Can you work these out from the model? Positions are in its coordinate system, mm. A direction names the side the tool comes from. Coordinates: 2 decimals unless noted, no trailing zeros. Loops run counter-clockwise (first coordinate to the right, second up) from the corner with the lowest first, then second, coordinate; pieces in that order, holes last.
```python
from build123d import *

# Parameters (mm, degrees)
ESQUISSE1_W             = 10
ESQUISSE1_H             = 15
BOSS_EXTRU_1_DEPTH      = 10
CONG_1_RADIUS           = 5
CONG_1_LENGTH           = 10
ESQUISSE3_W             = 5
ESQUISSE3_H             = 12
ENL_V_MAT_EXTRU_1_DEPTH = 10
ESQUISSE4_W             = 10
ESQUISSE4_H             = 10
BOSS_EXTRU_2_DEPTH      = 3
ESQUISSE5_R             = 1
ENL_V_MAT_EXTRU_2_DEPTH = 3
ESQUISSE6_R             = 2
ENL_V_MAT_EXTRU_3_DEPTH = 21.862646045
CONG_2_R                = 0.5
CONG_3_R                = 0.5


with BuildPart() as part:
    # Esquisse1 → Boss.-Extru.1 (new body)
    with BuildSketch(Plane.XY):
        Rectangle(ESQUISSE1_W, ESQUISSE1_H)
    extrude(amount=BOSS_EXTRU_1_DEPTH)

    # Congé1: full round fillet: the end face becomes a half cylinder, R = half its width
    cong_1_face = Plane((0, -7.5, 5), x_dir=(0, 0, 1), z_dir=(0, -1, 0))  # on the end face: x along it, z out of the body
    cong_1_slab = cong_1_face.offset(-CONG_1_RADIUS / 2) * Box(CONG_1_LENGTH, 2 * CONG_1_RADIUS, CONG_1_RADIUS, mode=Mode.PRIVATE)  # the body's end, R deep
    cong_1_round = Plane((0, -2.5, 5), x_dir=(0, -1, 0), z_dir=(0, 0, 1)) * Cylinder(CONG_1_RADIUS, CONG_1_LENGTH, mode=Mode.PRIVATE)  # its axis R under the face
    add(cong_1_slab - cong_1_round, mode=Mode.SUBTRACT)

    # Esquisse3 → Enlèv. mat.-Extru.1 (cut)
    with BuildSketch(Plane.ZY.offset(5)):
        with Locations((5, -1.5)):
            Rectangle(ESQUISSE3_W, ESQUISSE3_H)
    extrude(amount=-ENL_V_MAT_EXTRU_1_DEPTH, mode=Mode.SUBTRACT)

    # Esquisse4 → Boss.-Extru.2 (add)
    # profile 1 of 2: a face of its own
    with BuildSketch(Plane(origin=(0, 7.5, 0), x_dir=(1, 0, 0), z_dir=(0, 1, 0))):
        with BuildLine():
            Line((8, 5), (-8, 5))
            ThreePointArc((-8, 5), (-9.414213562, 4.414213562), (-10, 3))
            Line((-10, 3), (-10, -13))
            ThreePointArc((-10, -13), (-9.414213562, -14.414213562), (-8, -15))
            Line((-8, -15), (8, -15))
            ThreePointArc((8, -15), (9.414213562, -14.414213562), (10, -13))
            Line((10, -13), (10, 3))
            ThreePointArc((10, 3), (9.414213562, 4.414213562), (8, 5))
        make_face()
        with Locations((0, -5)):
            Rectangle(ESQUISSE4_W, ESQUISSE4_H, mode=Mode.SUBTRACT)
    # profile 2 of 2: a face of its own
    with BuildSketch(Plane(origin=(0, 7.5, 0), x_dir=(1, 0, 0), z_dir=(0, 1, 0))):
        with Locations((0, -5)):
            Rectangle(ESQUISSE4_W, ESQUISSE4_H)
    extrude(amount=BOSS_EXTRU_2_DEPTH)

    # Esquisse5 → Enlèv. mat.-Extru.2 (cut)
    with BuildSketch(Plane.XZ.offset(-7.5)):
        with Locations(Location((-7.5, 5, 0), (0, 0, 270))):
            Circle(ESQUISSE5_R)
        with Locations(Location((7.5, 5, 0), (0, 0, 270))):
            Circle(ESQUISSE5_R)
    extrude(amount=-ENL_V_MAT_EXTRU_2_DEPTH, mode=Mode.SUBTRACT)

    # Esquisse6 → Enlèv. mat.-Extru.3 (cut, through all)
    with BuildSketch(Plane.XY.offset(10)):
        with Locations((0, -2.5)):
            Circle(ESQUISSE6_R)
    extrude(amount=-ENL_V_MAT_EXTRU_3_DEPTH, mode=Mode.SUBTRACT)

    # Congé2
    cong_2_edges = [part.edges().sort_by_distance(p)[0] for p in [
        (-2, -2.5, 0),
        (-2, -2.5, 10),
    ]]
    fillet(cong_2_edges, radius=CONG_2_R)

    # Congé3
    cong_3_edges = [part.edges().sort_by_distance(p)[0] for p in [
        (0, 7.5, 0),
        (-5, 7.5, 5),
        (5, 7.5, 5),
        (0, 7.5, 10),
    ]]
    fillet(cong_3_edges, radius=CONG_3_R)


solid = part.part
```
(1) I want a section at A-A on y = 1.5. Write out the boundary of the cut face in (x, z), then the cut area to 3 significant figures.
Check values:
outline: (-5, 0) - (5, 0) - (5, 2.5) - (-5, 2.5) - close; (-5, 7.5) - (5, 7.5) - (5, 10) - (-5, 10) - close
area: 50.0 mm2
(2) I want a section at C-C on x = -7.5. Write out the boundary of the cut face in (y, z).
Check values:
outline: (7.5, -5) - (10.5, -5) - (10.5, 4) - (7.5, 4) - close; (7.5, 6) - (10.5, 6) - (10.5, 15) - (7.5, 15) - close
(3) I'm going to push flat-ended pins straight in: pin 1 (8 mm diameter, centred on x = 1, y = -3, fed in from +Z); pin 2 (8 mm diameter, centred on x = -2, y = -1, fed in from -Z); pin 3 (3 mm diameter, centred on x = -7.5, z = 5, fed in from -Y). Where does each tip first touch, or does it pass through?
Check values:
pin 1: stops at z = 10
pin 2: stops at z = 0
pin 3: stops at y = 7.5
(4) I want a section at B-B on z = 5. Write out the boundary of the cut face in (x, y).
Check values:
outline: (-10, 7.5) - (-8.5, 7.5) - (-8.5, 10.5) - (-10, 10.5) - close; (-6.5, 7.5) - (-5.5, 7.5) arc R0.5 cw to (-5, 7) - (-5, 4.5) - (5, 4.5) - (5, 7) arc R0.5 cw to (5.5, 7.5) - (6.5, 7.5) - (6.5, 10.5) - (-6.5, 10.5) - close; (8.5, 7.5) - (10, 7.5) - (10, 10.5) - (8.5, 10.5) - close
(5) I want a section at D-D on x = 0. Write out the boundary of the cut face in (y, z).
Check values:
outline: (-7.5, 0) - (-5, 0) arc R0.5 ccw to (-4.5, 0.5) - (-4.5, 2.5) - (-7.5, 2.5) - close; (-7.5, 7.5) - (-4.5, 7.5) - (-4.5, 9.5) arc R0.5 ccw to (-5, 10) - (-7.5, 10) - close; (-0.5, 0.5) arc R0.5 ccw to (0, 0) - (7, 0) arc R0.5 cw to (7.5, -0.5) - (7.5, -5) - (10.5, -5) - (10.5, 15) - (7.5, 15) - (7.5, 10.5) arc R0.5 cw to (7, 10) - (0, 10) arc R0.5 ccw to (-0.5, 9.5) - (-0.5, 7.5) - (4.5, 7.5) - (4.5, 2.5) - (-0.5, 2.5) - close
(6) Which directions (+Z, -Z, +X, -X, +Y, -Y) give clear straight access to the entire face, cutting with the end or side of a thin tool? Please do faces 4 (the flat face through (0, 1, 0)), 5 (the flat face through (0, 7.5, -2)), 6 (the flat face through (0, 1, 10)), 7 (the flat face through (5, 5, 5)).
Check values:
face 4: -Z, +X, -X, -Y
face 5: -Y
face 6: +Z, +X, -X, -Y
face 7: +Z, -Z, +X, -Y
(7) If we mould it in two halves opening along Y, with no side actions, what happens to faces 1 (the flat face through (0, 4.5, 5)), 2 (the cylindrical face through (-0.434, -4.452, 8.514)), 3 (the flat face through (-5, 5, 5))? For each: released by +Y, released by -Y, zero draft, split by the parting line, or undercut.
Check values:
face 1: released by -Y
face 2: undercut
face 3: zero draft
(8) If I drill on probe 1 along X at (y, z) = (9.15, 5); probe 2 along Z at (x, y) = (3.5, 2.5); probe 3 along Y at (x, z) = (0, 1.3), over which ranges is the centre line in solid material (lowest first)?
Check values:
probe 1: x = -10 to -8.5, -6.5 to 6.5, 8.5 to 10
probe 2: z = 0 to 2.5, 7.5 to 10
probe 3: y = -7.5 to -4.5, -0.5 to 10.5
